from build123d import *

# Parameters (mm, degrees)
BOSS_EXTRUDE5_DEPTH      = 3
BOSS_EXTRUDE5_DEPTH_BACK = 1
SKETCH2_W                = 80
SKETCH2_H                = 45.5
SKETCH2_R                = 2.5
SKETCH2_R_2              = 1.5
SKETCH2_R_3              = 4.25
SKETCH2_W_2              = 37.2
SKETCH2_H_2              = 4
SKETCH2_R_4              = 1.4
SKETCH2_8_R              = 2.5
SKETCH2_8_R_2            = 1.4
SKETCH2_8_W              = 37.2
SKETCH2_8_H              = 4
BOSS_EXTRUDE6_DEPTH      = 4.4
SKETCH7_R                = 1.45
CUT_EXTRUDE3_DEPTH       = 47.19050227
FILLET1_R                = 1


with BuildPart() as part:
    # Sketch2 → Boss-Extrude5 (new, two sides: drawn at the far end of the back side and taken through both)
    # profile 1 of 18: a face of its own
    with BuildSketch(Plane.XY.offset(-BOSS_EXTRUDE5_DEPTH_BACK)):
        Rectangle(SKETCH2_W, SKETCH2_H)
        with Locations((-8.718645076, -4.968645076)):
            Circle(SKETCH2_R, mode=Mode.SUBTRACT)
        with Locations((8.718645076, -4.968645076)):
            Circle(SKETCH2_R, mode=Mode.SUBTRACT)
        with Locations((8.718645076, 12.468645076)):
            Circle(SKETCH2_R, mode=Mode.SUBTRACT)
        with Locations((-8.718645076, 12.468645076)):
            Circle(SKETCH2_R, mode=Mode.SUBTRACT)
        with Locations((20, -19.25)):
            Circle(SKETCH2_R, mode=Mode.SUBTRACT)
        with Locations((-20, -19.25)):
            Circle(SKETCH2_R, mode=Mode.SUBTRACT)
        with Locations((20, 18.75)):
            Circle(SKETCH2_R, mode=Mode.SUBTRACT)
        with Locations((-20, 18.75)):
            Circle(SKETCH2_R, mode=Mode.SUBTRACT)
        with Locations((-37, 17.75)):
            Circle(SKETCH2_R_2, mode=Mode.SUBTRACT)
        with Locations((-37, -0.25)):
            Circle(SKETCH2_R_2, mode=Mode.SUBTRACT)
        with Locations((37, -0.25)):
            Circle(SKETCH2_R_2, mode=Mode.SUBTRACT)
        with Locations((37, 17.75)):
            Circle(SKETCH2_R_2, mode=Mode.SUBTRACT)
        with Locations((0, 3.75)):
            Circle(SKETCH2_R_3, mode=Mode.SUBTRACT)
        with Locations((-0.005934964, -9.695257034)):
            Rectangle(SKETCH2_W_2, SKETCH2_H_2, mode=Mode.SUBTRACT)
    # profile 2 of 18: a face of its own
    with BuildSketch(Plane.XY.offset(-BOSS_EXTRUDE5_DEPTH_BACK)):
        with Locations((-20, 18.75)):
            Circle(SKETCH2_R)
        with Locations((-20, 18.75)):
            Circle(SKETCH2_R_4, mode=Mode.SUBTRACT)
    # profile 3 of 18: a face of its own
    with BuildSketch(Plane.XY.offset(-BOSS_EXTRUDE5_DEPTH_BACK)):
        with Locations((-20, 18.75)):
            Circle(SKETCH2_R_4)
    # profile 4 of 18: a face of its own
    with BuildSketch(Plane.XY.offset(-BOSS_EXTRUDE5_DEPTH_BACK)):
        with Locations((-8.718645076, 12.468645076)):
            Circle(SKETCH2_R)
        with Locations((-8.718645076, 12.468645076)):
            Circle(SKETCH2_R_2, mode=Mode.SUBTRACT)
    # profile 5 of 18: a face of its own
    with BuildSketch(Plane.XY.offset(-BOSS_EXTRUDE5_DEPTH_BACK)):
        with Locations((-8.718645076, 12.468645076)):
            Circle(SKETCH2_R_2)
    # profile 6 of 18: a face of its own
    with BuildSketch(Plane.XY.offset(-BOSS_EXTRUDE5_DEPTH_BACK)):
        with Locations((8.718645076, 12.468645076)):
            Circle(SKETCH2_R)
        with Locations((8.718645076, 12.468645076)):
            Circle(SKETCH2_R_2, mode=Mode.SUBTRACT)
    # profile 7 of 18: a face of its own
    with BuildSketch(Plane.XY.offset(-BOSS_EXTRUDE5_DEPTH_BACK)):
        with Locations((8.718645076, 12.468645076)):
            Circle(SKETCH2_R_2)
    # profile 8 of 18: a face of its own
    with BuildSketch(Plane.XY.offset(-BOSS_EXTRUDE5_DEPTH_BACK)):
        with Locations((-8.718645076, -4.968645076)):
            Circle(SKETCH2_R)
        with Locations((-8.718645076, -4.968645076)):
            Circle(SKETCH2_R_2, mode=Mode.SUBTRACT)
    # profile 9 of 18: a face of its own
    with BuildSketch(Plane.XY.offset(-BOSS_EXTRUDE5_DEPTH_BACK)):
        with Locations((-8.718645076, -4.968645076)):
            Circle(SKETCH2_R_2)
    # profile 10 of 18: a face of its own
    with BuildSketch(Plane.XY.offset(-BOSS_EXTRUDE5_DEPTH_BACK)):
        with Locations((8.718645076, -4.968645076)):
            Circle(SKETCH2_R)
        with Locations((8.718645076, -4.968645076)):
            Circle(SKETCH2_R_2, mode=Mode.SUBTRACT)
    # profile 11 of 18: a face of its own
    with BuildSketch(Plane.XY.offset(-BOSS_EXTRUDE5_DEPTH_BACK)):
        with Locations((8.718645076, -4.968645076)):
            Circle(SKETCH2_R_2)
    # profile 12 of 18: a face of its own
    with BuildSketch(Plane.XY.offset(-BOSS_EXTRUDE5_DEPTH_BACK)):
        with Locations((20, 18.75)):
            Circle(SKETCH2_R)
        with Locations((20, 18.75)):
            Circle(SKETCH2_R_4, mode=Mode.SUBTRACT)
    # profile 13 of 18: a face of its own
    with BuildSketch(Plane.XY.offset(-BOSS_EXTRUDE5_DEPTH_BACK)):
        with Locations((20, 18.75)):
            Circle(SKETCH2_R_4)
    # profile 14 of 18: a face of its own
    with BuildSketch(Plane.XY.offset(-BOSS_EXTRUDE5_DEPTH_BACK)):
        with Locations((-0.005934964, -9.695257034)):
            Rectangle(SKETCH2_W_2, SKETCH2_H_2)
    # profile 15 of 18: a face of its own
    with BuildSketch(Plane.XY.offset(-BOSS_EXTRUDE5_DEPTH_BACK)):
        with Locations((20, -19.25)):
            Circle(SKETCH2_R)
        with Locations((20, -19.25)):
            Circle(SKETCH2_R_4, mode=Mode.SUBTRACT)
    # profile 16 of 18: a face of its own
    with BuildSketch(Plane.XY.offset(-BOSS_EXTRUDE5_DEPTH_BACK)):
        with Locations((20, -19.25)):
            Circle(SKETCH2_R_4)
    # profile 17 of 18: a face of its own
    with BuildSketch(Plane.XY.offset(-BOSS_EXTRUDE5_DEPTH_BACK)):
        with Locations((-20, -19.25)):
            Circle(SKETCH2_R)
        with Locations((-20, -19.25)):
            Circle(SKETCH2_R_4, mode=Mode.SUBTRACT)
    # profile 18 of 18: a face of its own
    with BuildSketch(Plane.XY.offset(-BOSS_EXTRUDE5_DEPTH_BACK)):
        with Locations((-20, -19.25)):
            Circle(SKETCH2_R_4)
    extrude(amount=BOSS_EXTRUDE5_DEPTH + BOSS_EXTRUDE5_DEPTH_BACK)

    # Sketch2<8> → Boss-Extrude6 (add)
    # profile 1 of 5: a face of its own
    with BuildSketch(Plane.XY):
        with Locations((20, 18.75)):
            Circle(SKETCH2_8_R)
        with Locations((20, 18.75)):
            Circle(SKETCH2_8_R_2, mode=Mode.SUBTRACT)
    # profile 2 of 5: a face of its own
    with BuildSketch(Plane.XY):
        with Locations((-20, 18.75)):
            Circle(SKETCH2_8_R)
        with Locations((-20, 18.75)):
            Circle(SKETCH2_8_R_2, mode=Mode.SUBTRACT)
    # profile 3 of 5: a face of its own
    with BuildSketch(Plane.XY):
        with Locations((-20, -19.25)):
            Circle(SKETCH2_8_R)
        with Locations((-20, -19.25)):
            Circle(SKETCH2_8_R_2, mode=Mode.SUBTRACT)
    # profile 4 of 5: a face of its own
    with BuildSketch(Plane.XY):
        with Locations((-0.005934964, -9.695257034)):
            Rectangle(SKETCH2_8_W, SKETCH2_8_H)
    # profile 5 of 5: a face of its own
    with BuildSketch(Plane.XY):
        with Locations((20, -19.25)):
            Circle(SKETCH2_8_R)
        with Locations((20, -19.25)):
            Circle(SKETCH2_8_R_2, mode=Mode.SUBTRACT)
    extrude(amount=-BOSS_EXTRUDE6_DEPTH)

    # Sketch7 → Cut-Extrude3 (cut, through all)
    with BuildSketch(Plane(origin=(0, 0, -1), x_dir=(-1, 0, 0), z_dir=(0, 0, -1))):
        with Locations((0, -4.125)):
            Circle(SKETCH7_R)
        with Locations((9.375, 3.75)):
            Circle(SKETCH7_R)
        with Locations((0, 11.625)):
            Circle(SKETCH7_R)
        with Locations((-9.375, 3.75)):
            Circle(SKETCH7_R)
    extrude(amount=-CUT_EXTRUDE3_DEPTH, mode=Mode.SUBTRACT)

    # Fillet1
    fillet1_edges = [part.edges().sort_by_distance(p)[0] for p in [
        (17.5, 18.75, -1),
        (-22.5, 18.75, -1),
        (-22.5, -19.25, -1),
        (17.5, -19.25, -1),
    ]]
    fillet(fillet1_edges, radius=FILLET1_R - 0.0001)  # a hair under: the kernel refuses the full size


solid = part.part
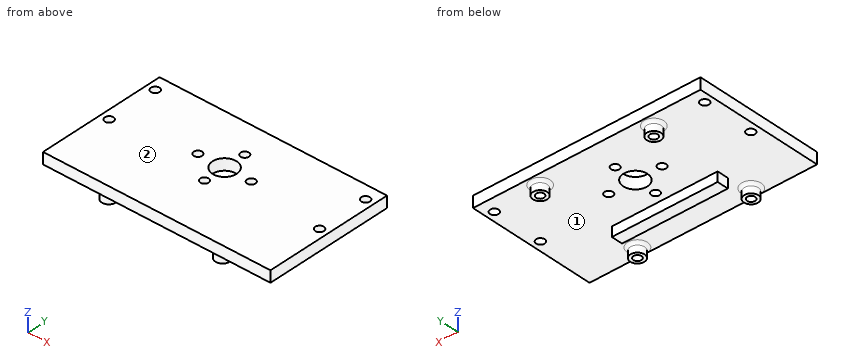
Check sheet for the modelled part. Datum: model origin and axes. Units: mm. Face numbers are marked on the shaded views. Round coordinates to 2 decimals unless told otherwise and drop trailing zeros. Order: outer loops, then holes, each group sorted by start corner. A loop starts at its lowest first (then second) coordinate and runs counter-clockwise, first axis right, second up. Notation, with made-up numbers: M -21.75,26 L 22.25,26 A27 cw 22.25,56 Z; hole C 82,33 d7. An arc over 180 degrees is marked long. One line per item, written item: value. Start each with the question number.
1. Gauge pin test, flat ends, axial feed: P1, Ø1, axis at x = 7.5, z = -3, coming from the +Y side; P2, Ø8, axis at x = -28.5, y = 8.5, coming from the -Z side; P3, Ø2.5, axis at y = -9.5, z = -3, coming from the -X side; P4, Ø2.5, axis at x = -37, y = -0.25, coming from the -Z side. Record the tip position at first contact, or that the pin passes through.
2. Section check B-B on x = -37. Enter the section's corners in (y, z).
3. Section check A-A on y = 3.75. Enter the section's corners in (x, z) (3 decimals).
4. Release check for a two-part mould opening along X. For the marked faces 1 and 2 record: released by +X, released by -X, zero draft, split by the parting line, or undercut.
5. Scan lines: line 1 along Y through (x, z) = (0, 1.6) (3 decimals); line 2 along Y through (x, z) = (37, 1.35); line 3 along Z through (x, y) = (-24, 3). Record each from-to range of solid material in increasing order.
6. Section check C-C on x = 0. Enter the section's corners in (y, z) (3 decimals).
7. Section check D-D on y = -19.25. Enter the section's corners in (x, z), and give its area (3 significant figures).
Results found:
1. P1: y = -7.7
1. P2: z = -1
1. P3: x = -18.61
1. P4: through
2. outline: M -22.75,-1 L -1.75,-1 L -1.75,3 L -22.75,3 Z; M 1.25,-1 L 16.25,-1 L 16.25,3 L 1.25,3 Z; M 19.25,-1 L 22.75,-1 L 22.75,3 L 19.25,3 Z
3. outline: M -40,-1 L -10.825,-1 L -10.825,3 L -40,3 Z; M -7.925,-1 L -4.25,-1 L -4.25,3 L -7.925,3 Z; M 4.25,-1 L 7.925,-1 L 7.925,3 L 4.25,3 Z; M 10.825,-1 L 40,-1 L 40,3 L 10.825,3 Z
4. face 1: undercut
4. face 2: zero draft
5. line 1: -22.75 to -5.575, -2.675 to -0.5, 8 to 10.175, 13.075 to 22.75
5. line 2: -22.75 to -1.75, 1.25 to 16.25, 19.25 to 22.75
5. line 3: -1 to 3
6. outline: M -22.75,-1 L -11.695,-1 L -11.695,-4.4 L -7.695,-4.4 L -7.695,-1 L -5.575,-1 L -5.575,3 L -22.75,3 Z; M -2.675,-1 L -0.5,-1 L -0.5,3 L -2.675,3 Z; M 8,-1 L 10.175,-1 L 10.175,3 L 8,3 Z; M 13.075,-1 L 22.75,-1 L 22.75,3 L 13.075,3 Z
7. outline: M -40,-1 L -23.5,-1 A1 cw -22.5,-2 L -22.5,-4.4 L -21.4,-4.4 L -21.4,-1 L -18.6,-1 L -18.6,-4.4 L -17.5,-4.4 L -17.5,-2 A1 cw -16.5,-1 L 16.5,-1 A1 cw 17.5,-2 L 17.5,-4.4 L 18.6,-4.4 L 18.6,-1 L 21.4,-1 L 21.4,-4.4 L 22.5,-4.4 L 22.5,-2 A1 cw 23.5,-1 L 40,-1 L 40,3 L -40,3 Z
7. area: 336 mm^2
